```python
from build123d import *

# Parameters (mm, degrees)
SKETCH1_W           = 140
SKETCH1_H           = 90
SKETCH1_W_2         = 105
SKETCH1_H_2         = 67
BOSS_EXTRUDE1_DEPTH = 2
SKETCH2_R           = 1.5
CUT_EXTRUDE1_DEPTH  = 89.602535605
CHAMFER1_SIZE       = 1.86
SKETCH8_W           = 117.8
SKETCH8_H           = 1
BOSS_EXTRUDE3_DEPTH = 1


with BuildPart() as part:
    # Sketch1 → Boss-Extrude1 (new body)
    with BuildSketch(Plane.XY):
        with Locations((1.473041333, -7.32603251)):
            Rectangle(SKETCH1_W, SKETCH1_H)
        with Locations((1.473041333, 0.17396749)):
            Rectangle(SKETCH1_W_2, SKETCH1_H_2, mode=Mode.SUBTRACT)
    extrude(amount=BOSS_EXTRUDE1_DEPTH)

    # Sketch2 → Cut-Extrude1 (cut, through all)
    with BuildSketch(Plane(origin=(0, 0, 0), x_dir=(-1, 0, 0), z_dir=(0, 0, -1))):
        with Locations((62.026958667, -37.82603251)):
            Circle(SKETCH2_R)
        with Locations((63.526958667, 24.67396749)):
            Circle(SKETCH2_R)
        with Locations((-64.973041333, -37.82603251)):
            Circle(SKETCH2_R)
        with Locations((-66.473041333, 24.67396749)):
            Circle(SKETCH2_R)
    extrude(amount=-CUT_EXTRUDE1_DEPTH, mode=Mode.SUBTRACT)

    # Chamfer1
    chamfer1_edges = [part.edges().sort_by_distance(p)[0] for p in [
        (-60.526958667, -37.82603251, 2),
        (-62.026958667, 24.67396749, 2),
        (66.473041333, -37.82603251, 2),
        (67.973041333, 24.67396749, 2),
    ]]
    chamfer(chamfer1_edges, length=CHAMFER1_SIZE)

    # Sketch8 → Boss-Extrude3 (add)
    with BuildSketch(Plane(origin=(0, 0, 0), x_dir=(-1, 0, 0), z_dir=(0, 0, -1))):
        with Locations((-1.473041333, -49.72603251)):
            Rectangle(SKETCH8_W, SKETCH8_H)
        with Locations((-1.473041333, 35.07396749)):
            Rectangle(SKETCH8_W, SKETCH8_H)
    extrude(amount=BOSS_EXTRUDE3_DEPTH)


solid = part.part
```
Part model, mm, in its own coordinate system. Round coordinates to 2 decimals unless told otherwise and drop trailing zeros. Write each loop counter-clockwise with the first axis right and the second up, starting at its lowest first coordinate (ties: lowest second). Pieces come first, ordered by that corner, then holes. Notation, with made-up numbers: M -34.5,-20 L -21.5,-20 A15 ccw -21.5,-13 Z; hole C 75,-34 d6. An arc over 180 degrees is marked long. One line per question, with ' | ' between items.
(1) Pin check, flat tips, straight feed: pin 1 (0.5 mm diameter, centred on x = -27.5, z = -0.5, fed in from +Y); pin 2 (0.8 mm diameter, centred on x = 14.5, z = -0.5, fed in from -Y); pin 3 (2.5 mm diameter, centred on x = -63.53, y = 24.67, fed in from +Z); pin 4 (1.1 mm diameter, centred on y = 35, z = -0.5, fed in from -X). Stop position of each tip, or through.
Answer key:
pin 1: stops at y = 35.57 | pin 2: stops at y = -50.23 | pin 3: passes through | pin 4: stops at x = -68.53
(2) Saw through at B-B on y = -6. Write the cut outline in (x, z).
Answer key:
outline: M -68.53,0 L -51.03,0 L -51.03,2 L -68.53,2 Z; M 53.97,0 L 71.47,0 L 71.47,2 L 53.97,2 Z
(3) Saw through at A-A on z = -0.55. Write the cut outline in (x, y), then the cut area to 3 significant figures.
Answer key:
outline: M -57.43,-50.23 L 60.37,-50.23 L 60.37,-49.23 L -57.43,-49.23 Z; M -57.43,34.57 L 60.37,34.57 L 60.37,35.57 L -57.43,35.57 Z | area: 236 mm^2
(4) Two-plate mould, pull along Y, no slides. Class faces 1 (the face through (0, -37, 0)), 2 (the face through (1, -34, 2)): released by +Y, released by -Y, zero draft, split by the parting line, or undercut.
Answer key:
face 1: undercut | face 2: zero draft
(5) Probe line 1 along Y through (x, z) = (-26.5, 1.15); line 2 along X through (y, z) = (7.5, 0.55); line 3 along Y through (x, z) = (16, -0.9). List the from-to ranges inside material, lowest first.
Answer key:
line 1: y = -52.33 to -33.33, 33.67 to 37.67 | line 2: x = -68.53 to -51.03, 53.97 to 71.47 | line 3: y = -50.23 to -49.23, 34.57 to 35.57
(6) Saw through at C-C on x = 50. Write the cut outline in (y, z).
Answer key:
outline: M -52.33,0 L -50.23,0 L -50.23,-1 L -49.23,-1 L -49.23,0 L -33.33,0 L -33.33,2 L -52.33,2 Z; M 33.67,0 L 34.57,0 L 34.57,-1 L 35.57,-1 L 35.57,0 L 37.67,0 L 37.67,2 L 33.67,2 Z
